from build123d import *

# Parameters (mm, degrees)
SKETCH5_W                            = 56
SKETCH5_H                            = 17
BOSS_EXTRUDE1_DEPTH                  = 22
F_10_0_10_DIAMETER_HOLE1_D           = 10
F_10_0_10_DIAMETER_HOLE1_CSINK_D     = 10.05
F_10_0_10_DIAMETER_HOLE1_CSINK_ANGLE = 90
FILLET1_R                            = 3
SKETCH10_R                           = 18.5
BOSS_EXTRUDE2_DEPTH                  = 40
F_20_0_20_DIAMETER_HOLE1_D           = 20
F_20_0_20_DIAMETER_HOLE1_CSINK_D     = 20.05
F_20_0_20_DIAMETER_HOLE1_CSINK_ANGLE = 90


with BuildPart() as part:
    # Sweep1: sweep along a path in Sketch2
    with BuildLine(Plane.XY) as sweep1_path:
        Line((-32, 0), (-32, 87))
        ThreePointArc((-32, 87), (-30.535533906, 90.535533906), (-27, 92))
        Line((-27, 92), (0, 92))
    # Sketch1 → Sweep1 (sweep)
    with BuildSketch(Plane(origin=(0, 0, 0), x_dir=(1, 0, 0), z_dir=(0, 1, 0))):
        Polygon((-32, 14), (-32, -14), (-40, -14), (-40, -4), (-62, -4), (-62, 4), (-40, 4), (-40, 14), align=None)
    sweep(path=sweep1_path.line)

    # Sketch5 → Boss-Extrude1 (add)
    with BuildSketch(Plane.ZY.offset(62)):
        with Locations((0, 8.5)):
            Rectangle(SKETCH5_W, SKETCH5_H)
    extrude(amount=-BOSS_EXTRUDE1_DEPTH)

    # Ø10.0 (10) Diameter Hole1 (through all)
    with Locations(Plane(origin=(-51, 17, 16), x_dir=(0, 0, 1), z_dir=(0, 1, 0))):
        with Locations((0, 0)):
            f_10_0_10_diameter_hole1 = CounterSinkHole(F_10_0_10_DIAMETER_HOLE1_D / 2, F_10_0_10_DIAMETER_HOLE1_CSINK_D / 2, counter_sink_angle=F_10_0_10_DIAMETER_HOLE1_CSINK_ANGLE)

    # Mirror1: Ø10.0 (10) Diameter Hole1 across plane
    add(f_10_0_10_diameter_hole1.mirror(Plane.XY), mode=Mode.SUBTRACT)

    # Fillet1
    fillet1_edges = [part.edges().sort_by_distance(p)[0] for p in [
        (-40, 8.5, -28),
        (-62, 8.5, -28),
        (-40, 8.5, 28),
        (-62, 8.5, 28),
    ]]
    fillet(fillet1_edges, radius=FILLET1_R)

    # Mirror2: part across plane


with BuildPart() as part_1:
    add(part.part)
    add(part.part.mirror(Plane(origin=(0, 0, 0), x_dir=(0, 0, 1), z_dir=(1, 0, 0))))

    # Sketch10 → Boss-Extrude2 (add)
    with BuildSketch(Plane(origin=(0, 125, 0), x_dir=(1, 0, 0), z_dir=(0, 1, 0))):
        with Locations(Location((0, 0, 0), (0, 0, 270))):
            Circle(SKETCH10_R)
    extrude(amount=-BOSS_EXTRUDE2_DEPTH)

    # Ø20.0 (20) Diameter Hole1 (through all)
    with Locations(Plane.ZX.offset(125)):
        with Locations((0, 0)):
            CounterSinkHole(F_20_0_20_DIAMETER_HOLE1_D / 2, F_20_0_20_DIAMETER_HOLE1_CSINK_D / 2, counter_sink_angle=F_20_0_20_DIAMETER_HOLE1_CSINK_ANGLE)


solid = part_1.part
Build history of the part. All positions in model axes, mm. A direction names the side the tool comes from. Round coordinates to 2 decimals unless told otherwise and drop trailing zeros. Loops run counter-clockwise (first coordinate to the right, second up) from the corner with the lowest first, then second, coordinate; pieces in that order, holes last. Notation, with made-up numbers: (83, -9.5) -> (125, -9.5) arc R17 cw to (125, 8.5) -> close; hole circle Ø9 at (-19.75, 88). An arc over 180 degrees is marked (long way). One line per item, written item: value. Start each with the question number.
Q1. Cut at D-D on x = 25.5. List the corners of the cut face in (y, z), plus the area to 3 significant figures.
Q2. Cut at C-C on x = -51. List the corners of the cut face in (y, z) (3 decimals).
Q3. Drop flat-ended pins along their axis: pin 1 Ø9 at (x, z) = (-24.5, -0.5) entering from +Y; pin 2 Ø14 at (x, y) = (27.5, 35) entering from -Z; pin 3 Ø6.5 at (x, z) = (-46, 15) entering from +Y; pin 4 Ø11.5 at (x, z) = (51, 16) entering from -Y. Give the stop position or say it passes through.
Q4. 3-axis set-ups, long thin cutter, end or side, ignore diameter. For faces 1 (the face through (-16.41, 105.28, 8.54)), 2 (the face through (51.2, 17, 21.2)), 3 (the face through (-40, 52, -9)): which of +Z, -Z, +X, -X, +Y, -Y reach the whole face in a straight line?
Q5. Cut at A-A on y = 80. List the corners of the cut face in (x, z).
Q6. Two-plate mould, pull along X, no slides. Class faces 4 (the face through (40, 52, 9)), 5 (the face through (40.9, 8.62, 27.14)), 6 (the face through (32, 44, 0)), 7 (the face through (-51, 8, -28)): released by +X, released by -X, zero draft, split by the parting line, or undercut.
Q7. Probe line 1 along X through (y, z) = (6, 16); line 2 along Z through (x, y) = (-51, 7); line 3 along X through (y, z) = (56, -0.5). List the from-to ranges inside material, lowest first.
Q8. Cut at B-B on z = 0. List the corners of the cut face in (x, y) (3 decimals).
Computed:
1. outline: (92, -14) -> (100, -14) -> (100, -4) -> (122, -4) -> (122, 4) -> (100, 4) -> (100, 14) -> (92, 14) -> close
1. area: 400 mm²
2. outline: (0, -28) -> (17, -28) -> (17, -21.025) -> (16.975, -21) -> (0, -21) -> close; (0, -11) -> (16.975, -11) -> (17, -10.975) -> (17, -4) -> (112.475, -4) -> (112.475, 4) -> (17, 4) -> (17, 10.975) -> (16.975, 11) -> (0, 11) -> close; (0, 21) -> (16.975, 21) -> (17, 21.025) -> (17, 28) -> (0, 28) -> close
3. pin 1: y = 122
3. pin 2: z = -14
3. pin 3: y = 17
3. pin 4: y = 0
4. face 1: none
4. face 2: +Z, +X, +Y
4. face 3: -Z, -X, +Y
5. outline: (-62, -4) -> (-40, -4) -> (-40, -14) -> (-32, -14) -> (-32, 14) -> (-40, 14) -> (-40, 4) -> (-62, 4) -> close; (32, -14) -> (40, -14) -> (40, -4) -> (62, -4) -> (62, 4) -> (40, 4) -> (40, 14) -> (32, 14) -> close
6. face 4: released by +X
6. face 5: undercut
6. face 6: undercut
6. face 7: zero draft
7. line 1: -62 to -56, -46 to -40, 40 to 46, 56 to 62
7. line 2: -28 to -21, -11 to 11, 21 to 28
7. line 3: -62 to -32, 32 to 62
8. outline: (-62, 0) -> (-32, 0) -> (-32, 87) arc R5 cw to (-27, 92) -> (-18.5, 92) -> (-18.5, 85) -> (-10, 85) -> (-10, 124.975) -> (-10.025, 125) -> (-18.5, 125) -> (-18.5, 122) -> (-27, 122) arc R35 ccw to (-62, 87) -> close; (10, 85) -> (18.5, 85) -> (18.5, 92) -> (27, 92) arc R5 cw to (32, 87) -> (32, 0) -> (62, 0) -> (62, 87) arc R35 ccw to (27, 122) -> (18.5, 122) -> (18.5, 125) -> (10.025, 125) -> (10, 124.975) -> close
